```python
from build123d import *

# Parameters (mm, degrees)
F1_W     = 25.4
F1_H     = 25.4
F2_DEPTH = 71.8312
F4_DEPTH = 25.4
F5_R     = 3.175


# Not quite as in the source:
# - a variable given as a bare number and used for a length is read in inches; the dataset says mm whatever the document's units were
# - a feature names something its author has since deleted; it is built from what else it names


with BuildPart() as f2:
    # F1 (on Top) → F2 (new body)
    with BuildSketch(Plane.XY):
        Rectangle(F1_W, F1_H)
        with BuildLine():
            ThreePointArc((-11.049, 7.874), (-10.1190640303, 10.1190640303), (-7.874, 11.049))
            Line((-7.874, 11.049), (7.874, 11.049))
            ThreePointArc((7.874, 11.049), (10.1190640303, 10.1190640303), (11.049, 7.874))
            Line((11.049, 7.874), (11.049, -7.874))
            ThreePointArc((11.049, -7.874), (10.1190640303, -10.1190640303), (7.874, -11.049))
            Line((7.874, -11.049), (-7.874, -11.049))
            ThreePointArc((-7.874, -11.049), (-10.1190640303, -10.1190640303), (-11.049, -7.874))
            Line((-11.049, -7.874), (-11.049, 7.874))
        make_face(mode=Mode.SUBTRACT)
    extrude(amount=F2_DEPTH)

    # F3 (on face) → F4 (cut)
    with BuildSketch(Plane.XZ.offset(12.7)):
        Polygon((12.7, 10.5210244843), (-12.7, 0), (12.7, 0), align=None)
        Polygon((12.7, 71.8312), (-12.7, 71.8312), (12.7, 61.3101755157), align=None)
    extrude(amount=-F4_DEPTH, mode=Mode.SUBTRACT)

    # F5
    f5_edges = [f2.edges().sort_by_distance(p)[0] for p in [
        (-12.7, 12.7, 35.9156),
        (12.7, 12.7, 35.9156),
        (-12.7, -12.7, 35.9156),
        (12.7, -12.7, 35.9156),
    ]]
    fillet(f5_edges, radius=F5_R)


solid = f2.part
```
Geometry: final body of the model. Coordinates: model frame, mm. A direction names the side the tool comes from. Coordinates: 2 decimals unless noted, no trailing zeros. Order: outer loops, then holes, each group sorted by start corner. A loop starts at its lowest first (then second) coordinate and runs counter-clockwise, first axis right, second up. Notation, with made-up numbers: (18.25, 21) - (70.25, 21) arc R30 ccw to (70.25, 56) - close; hole circle Ø4 at (38, 82.25). An arc over 180 degrees is marked (long way). Return JSON: item names as keys, results as strings. Group by question number.
1. Cut plane B-B (z = 58.5). Output: boundary loops of the cut face in (x, y) (3 decimals).
2. Cut plane C-C (x = -0.25). Output: boundary loops of the cut face in (y, z).
3. Pull-direction query (X, two-part tool) for faces 1 (the face through (-11.79, -11.75, 36.42)), 2 (the face through (0, 12.7, 35)), 3 (the face through (-11.049, 0, 35)); classes: pulls with the +X half, pulls with the -X half, needs draft (parallel to the pull), parting line crosses it, or undercut.
4. Set-up query: faces 4 (the face through (11.75, 11.79, 36.29)), 5 (the face through (10.094, 10.144, 35.532)). Return all of +Z, -Z, +X, -X, +Y, -Y with unobstructed straight access to the full face (end or side cutting, diameter ignored); none if empty.
5. Pin query (flat end, axial travel): pin 1 (4 mm diameter, centred on x = 8, y = 6, fed in from -Z); pin 2 (6 mm diameter, centred on x = -5, y = -8.5, fed in from -Z). Return the tip coordinate at first contact, or that it passes through.
6. Cut plane A-A (y = 4.5). Output: boundary loops of the cut face in (x, z).
7. Material intervals for line 1 along Y through (x, z) = (-6.25, 4.5); line 2 along X through (y, z) = (5, 63.5), sorted ascending. Write a range as [from, to].
Resolved:
{
 "1": {"outline": "(-12.7, -9.525) arc R3.175 ccw to (-9.525, -12.7) - (9.525, -12.7) arc R3.175 ccw to (12.7, -9.525) - (12.7, 9.525) arc R3.175 ccw to (9.525, 12.7) - (-9.525, 12.7) arc R3.175 ccw to (-12.7, 9.525) - close; hole (-11.049, -7.874) arc R3.175 ccw to (-7.874, -11.049) - (7.874, -11.049) arc R3.175 ccw to (11.049, -7.874) - (11.049, 7.874) arc R3.175 ccw to (7.874, 11.049) - (-7.874, 11.049) arc R3.175 ccw to (-11.049, 7.874) - close"},
 "2": {"outline": "(-12.7, 5.16) - (-11.05, 5.16) - (-11.05, 66.67) - (-12.7, 66.67) - close; (11.05, 5.16) - (12.7, 5.16) - (12.7, 66.67) - (11.05, 66.67) - close"},
 "3": {"face 1": "pulls with the -X half", "face 2": "needs draft", "face 3": "undercut"},
 "4": {"face 4": "+Z, -Z, +X, +Y", "face 5": "+Z, -Z"},
 "5": {"pin 1": "passes through", "pin 2": "stops at z = 2.53"},
 "6": {"outline": "(-12.7, 0) - (-11.05, 0.68) - (-11.05, 71.15) - (-12.7, 71.83) - close; (11.05, 9.84) - (12.7, 10.52) - (12.7, 61.31) - (11.05, 61.99) - close"},
 "7": {"line 1": "y = [-12.7, -11.05], [11.05, 12.7]", "line 2": "x = [-12.7, -11.05]"}
}
